Print and shaded views of the part. All mm, measured from the part's lowest x, y and z. Give positions to 0.01 mm unless a question says otherwise; leave off trailing zeros. Loops run counter-clockwise (first coordinate to the right, second up) from the corner with the lowest first, then second, coordinate; pieces in that order, holes last. Notation, with made-up numbers: M -1.5,5 L 34.5,5 A16 cw 34.5,29 Z; hole C 65,49.25 d4. An arc over 180 degrees is marked long. Put each result on its own line as item: value. Start each with the question number.
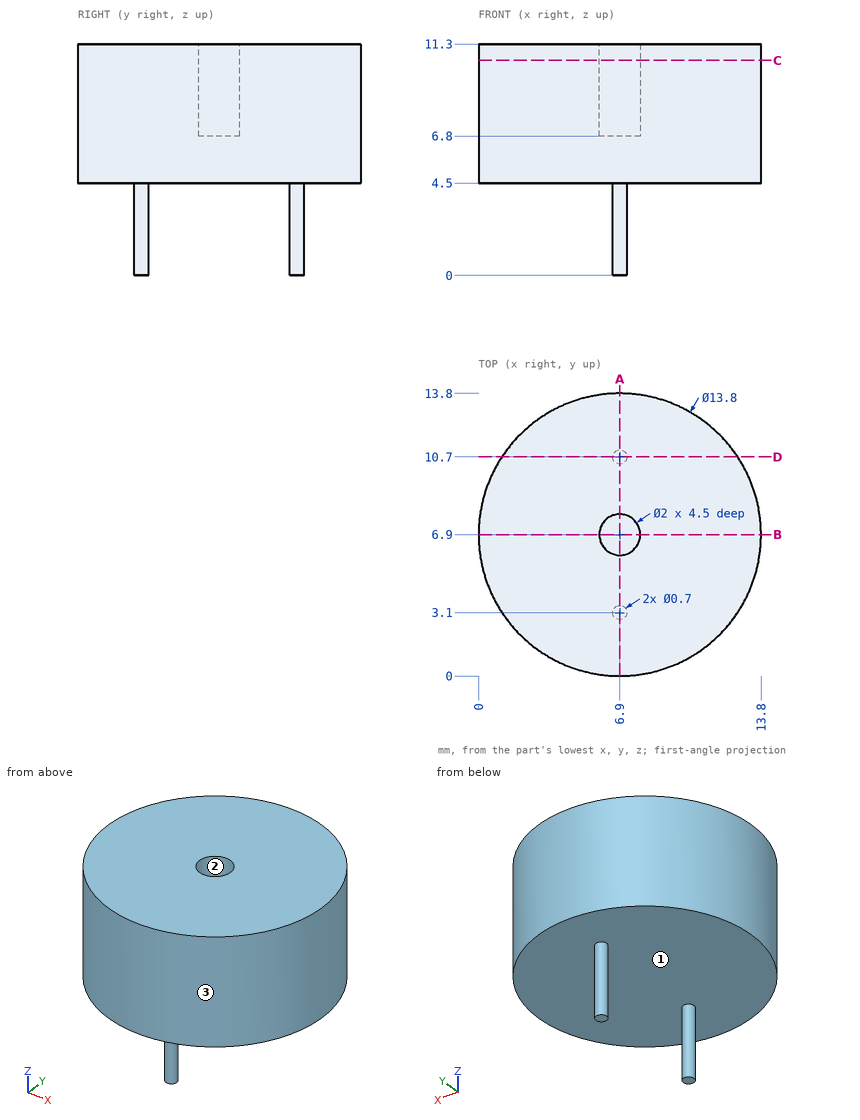
1) Mould opens along X. For the marked faces 1, 2 and 3 say: +X half, -X half, draft (parallel to the pull), parting line (faces both ways), or undercut.
2) Band-saw the part on B-B on y = 6.9. Give the cut face in (x, z), then the cut area to 3 significant figures.
3) Band-saw the part on D-D on y = 10.7. Give the cut face in (x, z).
4) Band-saw the part on C-C on z = 10.5. Give the cut face in (x, y).
5) Band-saw the part on A-A on x = 6.9. Give the cut face in (y, z), then the cut area to 3 significant figures.
6) Pin check, flat tips, straight feed: pin 1 Ø3 at (y, z) = (10, 9.5) entering from +X; pin 2 Ø6 at (x, z) = (12, 5) entering from +Y; pin 3 Ø1.5 at (x, z) = (5, 3) entering from -Y; pin 4 Ø4 at (x, y) = (4, 5) entering from -Z. Stop position of each tip, or through.
7) Wall check: L1, parallel to Y at x = 6.9, z = 8.35; L2, parallel to Z at x = 11.75, y = 2.5; L3, parallel to Y at x = 7.5, z = 9.75. Give the ranges that are in metal, low to high.
Evaluation:
1. face 1: draft
1. face 2: undercut
1. face 3: parting line
2. outline: M 0,4.5 L 13.8,4.5 L 13.8,11.3 L 7.9,11.3 L 7.9,6.8 L 5.9,6.8 L 5.9,11.3 L 0,11.3 Z
2. area: 84.8 mm2
3. outline: M 1.14,4.5 L 6.55,4.5 L 6.55,0 L 7.25,0 L 7.25,4.5 L 12.66,4.5 L 12.66,11.3 L 1.14,11.3 Z
4. outline: C 6.9,6.9 d13.8; hole C 6.9,6.9 d2
5. outline: M 0,4.5 L 2.75,4.5 L 2.75,0 L 3.45,0 L 3.45,4.5 L 10.35,4.5 L 10.35,0 L 11.05,0 L 11.05,4.5 L 13.8,4.5 L 13.8,11.3 L 7.9,11.3 L 7.9,6.8 L 5.9,6.8 L 5.9,11.3 L 0,11.3 Z
5. area: 91.1 mm2
6. pin 1: x = 13.61
6. pin 2: y = 13.47
6. pin 3: through
6. pin 4: z = 4.5
7. L1: 0 to 5.9, 7.9 to 13.8
7. L2: 4.5 to 11.3
7. L3: 0.03 to 6.1, 7.7 to 13.77
